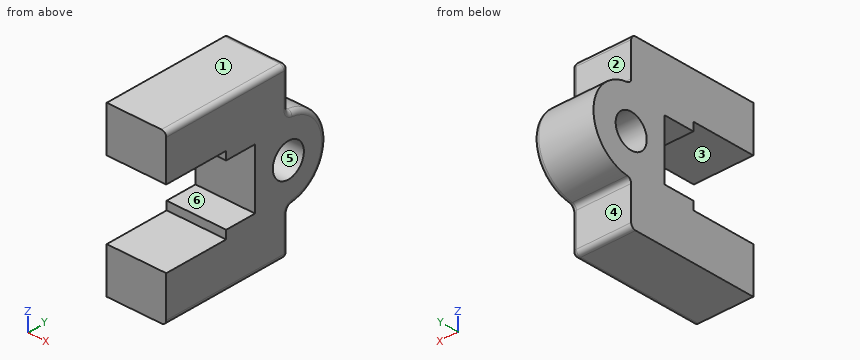
from build123d import *

# Parameters (mm, degrees)
SKETCH1_R           = 7
BOSS_EXTRUDE1_DEPTH = 25
CUT_EXTRUDE1_DEPTH  = 84.868945385
FILLET1_R           = 2
FILLET2_R           = 2


with BuildPart() as part:
    # Sketch1 → Boss-Extrude1 (new body)
    with BuildSketch(Plane(origin=(0, 0, 0), x_dir=(0, 0, -1), z_dir=(1, 0, 0))):
        with BuildLine():
            Line((17, 55), (35, 55))
            Line((35, 55), (35, 0))
            Line((35, 0), (-35, 0))
            Line((-35, 0), (-35, 55))
            Line((-35, 55), (-17, 55))
            ThreePointArc((-17, 55), (0, 72), (17, 55))
        make_face()
        with Locations((0, 55)):
            Circle(SKETCH1_R, mode=Mode.SUBTRACT)
    extrude(amount=BOSS_EXTRUDE1_DEPTH)

    # Sketch2 → Cut-Extrude1 (cut, through all)
    with BuildSketch(Plane(origin=(25, 0, 0), x_dir=(0, 0, -1), z_dir=(1, 0, 0))):
        Polygon((-16, 27), (-12.5, 27), (-12.5, 40), (12.5, 40), (12.5, 27), (16, 27), (16, 0), (-16, 0), align=None)
    extrude(amount=-CUT_EXTRUDE1_DEPTH, mode=Mode.SUBTRACT)

    # Fillet1
    fillet1_edges = [part.edges().sort_by_distance(p)[0] for p in [
        (12.5, 55, 35),
        (12.5, 55, 17),
        (12.5, 55, -17),
        (12.5, 55, -35),
    ]]
    fillet(fillet1_edges, radius=FILLET1_R)

    # Fillet2
    fillet2_edges = [part.edges().sort_by_distance(p)[0] for p in [
        (25, 26.5, -35),
        (25, 55, -25.947221814),
        (25, 72, 0),
        (25, 55, 25.947221814),
        (25, 26.5, 35),
        (25, 54.414213562, 34.414213562),
        (25, 54.414213562, -34.414213562),
        (25, 55.513216117, -17.55673152),
        (25, 55.513216117, 17.55673152),
    ]]
    fillet(fillet2_edges, radius=FILLET2_R)


solid = part.part
Design review of the part built by this model. Coordinates are the model's own, in mm. Face numbers are marked on the shaded views. A direction names the side the tool comes from. Coordinates: 2 decimals unless noted, no trailing zeros. Order: outer loops, then holes, each group sorted by start corner. A loop starts at its lowest first (then second) coordinate and runs counter-clockwise, first axis right, second up. Notation, with made-up numbers: (85, 16.5) -> (106, 16.5) arc R16 cw to (106, 47.5) -> close; hole circle Ø8 at (77.25, 46). An arc over 180 degrees is marked (long way). Use one line per item in the form item = value. Start each with the question number.
(1) Add section B-B on x = 11.25. State the section outline as (y, z) points.
(2) The part is to be moulded in two halves that separate along Z. For the marked faces 1, 2 and 3, say which applies: +Z half, -Z half, draft (parallel to the pull), parting line (faces both ways), or undercut.
(3) For probe 1 along Z at (x, y) = (8.5, 33); probe 2 along Y at (x, z) = (19, 0); probe 3 along Z at (x, y) = (2.5, 15.5), list the stretches that pass through material, from the lowest coordinate up.
(4) Add section D-D on y = 49.5. State the section outline as (x, z) points.
(5) Add section C-C on z = 0. State the section outline as (x, y) points.
(6) Insertion check: pin 1 (5 mm diameter, centred on y = 14, z = 25, fed in from -X); pin 2 (6 mm diameter, centred on y = 34.5, z = 8, fed in from +X); pin 3 (4 mm diameter, centred on x = 15, z = -24, fed in from +Y); pin 4 (1 mm diameter, centred on x = 18.5, z = -13.5, fed in from -Y). Each pin has a flat end and moves straight along its axis. Give the tip position at first contact, or say it passes through.
(7) For the marked faces 4, 5 and 6, list the 3-axis set-ups (+Z, -Z, +X, -X, +Y, -Y) from which the entire face can be reached by the end or side of a thin tool; tool diameter is ignored.
(8) Add section A-A on y = 7. State the section outline as (x, z) points, plus the area to 3 significant figures.
Answer block:
q1.outline = (0, -35) -> (53, -35) arc R2 ccw to (55, -33) -> (55, -18.89) arc R2 cw to (56.79, -16.91) arc R17 ccw to (56.79, 16.91) arc R2 cw to (55, 18.89) -> (55, 33) arc R2 ccw to (53, 35) -> (0, 35) -> (0, 16) -> (27, 16) -> (27, 12.5) -> (40, 12.5) -> (40, -12.5) -> (27, -12.5) -> (27, -16) -> (0, -16) -> close; hole circle Ø14 at (55, 0)
q2.face_1 = +Z half
q2.face_2 = draft
q2.face_3 = undercut
q3.probe_1 = -35 to -12.5, 12.5 to 35
q3.probe_2 = 40 to 48, 62 to 72
q3.probe_3 = -35 to -16, 16 to 35
q4.outline = (0, -35) -> (23, -35) arc R2 ccw to (25, -33) -> (25, -4.33) -> (0, -4.33) -> close; (0, 4.33) -> (25, 4.33) -> (25, 33) arc R2 ccw to (23, 35) -> (0, 35) -> close
q5.outline = (0, 40) -> (25, 40) -> (25, 48) -> (0, 48) -> close; (0, 62) -> (25, 62) -> (25, 70) arc R2 ccw to (23, 72) -> (0, 72) -> close
q6.pin_1 = 0
q6.pin_2 = through
q6.pin_3 = 55
q6.pin_4 = 27
q7.face_4 = -Z, +X, -X, +Y
q7.face_5 = +X, -X
q7.face_6 = +X, -X, -Y
q8.outline = (0, -35) -> (23, -35) arc R2 ccw to (25, -33) -> (25, -16) -> (0, -16) -> close; (0, 16) -> (25, 16) -> (25, 33) arc R2 ccw to (23, 35) -> (0, 35) -> close
q8.area = 948 mm²
